```python
from build123d import *

# Parameters (mm, degrees)
F1_DEPTH  = 4
F0_W      = 107
F0_H      = 2.5
F2_DEPTH  = 33
F3_W      = 20
F3_H      = 19.215
F3_R      = 2.2232187412
F4_DEPTH  = 2
F6_D      = 4
F6_DEPTH  = 12
F6_TIP    = 1.2017212381
F7_D      = 4
F8_DEPTH  = 10
F9_F1_R   = 1.9313708499
F9_F2_R   = 1.9313708499
F10_W     = 15
F10_H     = 10
F11_DEPTH = 11.3
F0_W_2    = 2.4193752706
F0_H_2    = 9.5048956573
F0_W_3    = 2.649404496
F0_H_3    = 10.744664818
F12_DEPTH = 25
F13_R     = 1.2071067812


with BuildPart() as f1:
    # F0 (on Top) → F1 (new body)
    with BuildSketch(Plane.XY):
        Polygon((-53.5, -35), (53.5, -35), (53.5, -5.4848068394), (53.5, 5.2598579787), (53.5, 35), (-53.5, 35), (-53.5, 25.9394217283), (-53.5, 16.434526071), (-53.5, -16.434526071), (-53.5, -25.9394217283), align=None)
        with BuildLine():
            Line((38.5, 24), (38.5, -24))
            Line((38.5, -24), (7.5, -24))
            ThreePointArc((7.5, -24), (1.5, -19), (-4.5, -24))
            Line((-4.5, -24), (-38.5, -24))
            Line((-38.5, -24), (-38.5, 24))
            Line((-38.5, 24), (-4.5, 24))
            ThreePointArc((-4.5, 24), (1.5, 19), (7.5, 24))
            Line((7.5, 24), (38.5, 24))
        make_face(mode=Mode.SUBTRACT)
    extrude(amount=F1_DEPTH)

    # F0 (on Top) → F2 (join)
    with BuildSketch(Plane.XY):
        with Locations((0, 36.25)):
            Rectangle(F0_W, F0_H)
        with Locations((0, -36.25)):
            Rectangle(F0_W, F0_H)
    extrude(amount=F2_DEPTH)

    # F3 (on face) → F4 (join)
    with BuildSketch(Plane.XY):
        with Locations((-37.3952314258, -44.6075)):
            Rectangle(F3_W, F3_H)
        with Locations((-37.3952314258, -41.215)):
            Circle(F3_R, mode=Mode.SUBTRACT)
        with Locations((37.3952314258, -44.6075)):
            Rectangle(F3_W, F3_H)
        with Locations((37.3952314258, -41.215)):
            Circle(F3_R, mode=Mode.SUBTRACT)
        with Locations((37.3952314258, 44.6075)):
            Rectangle(F3_W, F3_H)
        with Locations((37.3952314258, 41.215)):
            Circle(F3_R, mode=Mode.SUBTRACT)
        with Locations((-37.3952314258, 44.6075)):
            Rectangle(F3_W, F3_H)
        with Locations((-37.3952314258, 41.215)):
            Circle(F3_R, mode=Mode.SUBTRACT)
    extrude(amount=F4_DEPTH)

    # F6
    with Locations(Plane(origin=(0, 37.5, 0), x_dir=(-1, 0, 0), z_dir=(0, 1, 0))):
        with Locations((43.5, 23)):
            Hole(F6_D / 2, depth=F6_DEPTH)
            with Locations((0, 0, -(F6_DEPTH + F6_TIP / 2))):  # 118° drill point
                Cone(0, F6_D / 2, F6_TIP, mode=Mode.SUBTRACT)

    # F7 (through all)
    with Locations(Plane(origin=(0, 37.5, 0), x_dir=(-1, 0, 0), z_dir=(0, 1, 0))):
        with Locations((0, 16.522007063)):
            Hole(F7_D / 2)

    # F0 (on Top) → F8 (join)
    with BuildSketch(Plane.XY):
        with BuildLine():
            Line((7.5, -24), (38.5, -24))
            Line((38.5, -24), (38.5, 24))
            Line((38.5, 24), (7.5, 24))
            ThreePointArc((7.5, 24), (1.5, 19), (-4.5, 24))
            Line((-4.5, 24), (-38.5, 24))
            Line((-38.5, 24), (-38.5, -24))
            Line((-38.5, -24), (-4.5, -24))
            ThreePointArc((-4.5, -24), (1.5, -19), (7.5, -24))
        make_face()
    extrude(amount=F8_DEPTH)

    # F9: fillet of radius 1.9313708499 on 12 edges, made by hand

    # F9_f1
    f9_f1_edges = [f1.edges().sort_by_distance(p)[0] for p in [
        (0, -35, 4),
        (0, 35, 4),
        (1.5, 19, 4),
        (23, 24, 4),
        (38.5, 0, 4),
        (23, -24, 4),
        (1.5, -19, 4),
        (-21.5, -24, 4),
        (-38.5, 0, 4),
        (-21.5, 24, 4),
    ]]
    fillet(f9_f1_edges, radius=F9_F1_R)

    # F9_f2
    f9_f2_edges = [f1.edges().sort_by_distance(p)[0] for p in [
        (53.5, 0, 4),
        (-53.5, 0, 4),
        (-53.5, -34.4343145751, 4.5656854249),
        (-53.5, 34.4343145751, 4.5656854249),
        (53.5, 34.4343145751, 4.5656854249),
        (53.5, -34.4343145751, 4.5656854249),
    ]]
    fillet(f9_f2_edges, radius=F9_F2_R)

    # F10 (on face) → F11 (cut)
    with BuildSketch(Plane.XY):
        with Locations((-46.3137403131, 0)):
            Rectangle(F10_W, F10_H)
    extrude(amount=F11_DEPTH, mode=Mode.SUBTRACT)

    # F0 (on Top) → F12 (join)
    with BuildSketch(Plane.XY):
        with Locations((-54.7096876353, 21.1869738996)):
            Rectangle(F0_W_2, F0_H_2)
        with Locations((-54.7096876353, -21.1869738996)):
            Rectangle(F0_W_2, F0_H_2)
        with Locations((54.824702248, -0.1124744304)):
            Rectangle(F0_W_3, F0_H_3)
    extrude(amount=F12_DEPTH)

    # F13
    f13_edges = [f1.edges().sort_by_distance(p)[0] for p in [
        (-55.919375, 25.939422, 12.5),
        (-55.919375, 16.434526, 12.5),
        (-55.919375, 21.186974, 0),
        (-55.919375, 21.186974, 25),
        (-55.919375, -16.434526, 12.5),
        (-55.919375, -25.939422, 12.5),
        (-55.919375, -21.186974, 0),
        (-55.919375, -21.186974, 25),
        (56.149404, -5.484807, 12.5),
        (56.149404, 5.259858, 12.5),
        (56.149404, -0.112474, 0),
        (56.149404, -0.112474, 25),
    ]]
    fillet(f13_edges, radius=F13_R)


solid = f1.part
```
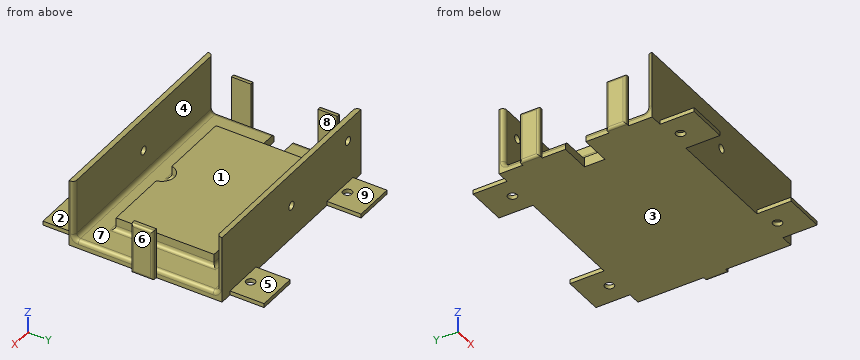
Model file for the job. Use its own axes, mm. Face numbers are marked on the shaded views. A direction names the side the tool comes from. Coordinates: 2 decimals unless noted, no trailing zeros. Loops run counter-clockwise (first coordinate to the right, second up) from the corner with the lowest first, then second, coordinate; pieces in that order, holes last. Notation, with made-up numbers: (-31.75, 58) -> (-25.75, 58) arc R28 cw to (-25.75, 85) -> close; hole circle Ø1 at (27, 40). An arc over 180 degrees is marked (long way). Answer as a JSON object with one key per item and string values.
Q1. Cut at C-C (x = 44). List the corners of the cut face in (y, z) (3 decimals), and give its area (3 significant figures).
Report:
{"outline": "(-54.215, 0) -> (54.215, 0) -> (54.215, 2) -> (37.5, 2) -> (37.5, 33) -> (35, 33) -> (35, 5.931) arc R1.931 cw to (33.069, 4) -> (-33.069, 4) arc R1.931 cw to (-35, 5.931) -> (-35, 33) -> (-37.5, 33) -> (-37.5, 2) -> (-54.215, 2) -> close", "area": "513 mm2"}
Q2. Cut at B-B (y = -11). List the corners of the cut face in (x, z).
Report:
{"outline": "(-53.5, 0) -> (53.5, 0) -> (53.5, 2.07) arc R1.93 ccw to (51.57, 4) -> (40.43, 4) arc R1.93 cw to (38.5, 5.93) -> (38.5, 10) -> (-38.5, 10) -> (-38.5, 5.93) arc R1.93 cw to (-40.43, 4) -> (-51.57, 4) arc R1.93 ccw to (-53.5, 2.07) -> close"}
Q3. Cut at A-A (x = -43.5). List the corners of the cut face in (y, z) (3 decimals), and give its area (3 significant figures).
Report:
{"outline": "(-54.215, 0) -> (-5, 0) -> (-5, 4) -> (-33.069, 4) arc R1.931 cw to (-35, 5.931) -> (-35, 33) -> (-37.5, 33) -> (-37.5, 2) -> (-54.215, 2) -> close; (5, 0) -> (54.215, 0) -> (54.215, 2) -> (37.5, 2) -> (37.5, 21) -> (35, 21) -> (35, 5.931) arc R1.931 cw to (33.069, 4) -> (5, 4) -> close; (35, 25) -> (37.5, 25) -> (37.5, 33) -> (35, 33) -> close", "area": "463 mm2"}
Q4. 3-axis set-ups, long thin cutter, end or side, ignore diameter. For the marked faces 1, 2, 3, 4 and 5: which of +Z, -Z, +X, -X, +Y, -Y reach the whole face in a straight line?
Report:
{"face 1": "+Z", "face 2": "+Z, +X, -X, -Y", "face 3": "-Z, +X, -X, +Y, -Y", "face 4": "+Z, +X, -X", "face 5": "+Z, +X, -X, +Y"}
Q5. Pull direction X, two halves, no side cores. Call the marked faces 6, 7, 8 and 9: released by +X, released by -X, zero draft, split by the parting line, or undercut.
Report:
{"face 6": "released by +X", "face 7": "undercut", "face 8": "undercut", "face 9": "zero draft"}
Q6. Cut at D-D (y = -31). List the corners of the cut face in (x, z), and give its area (3 significant figures).
Report:
{"outline": "(-53.5, 0) -> (53.5, 0) -> (53.5, 2.07) arc R1.93 ccw to (51.57, 4) -> (-51.57, 4) arc R1.93 ccw to (-53.5, 2.07) -> close", "area": "426 mm2"}
Q7. Probe probe 1 along Y at (x, z) = (-38.5, 11.5); probe 2 along X at (y, z) = (-17.5, 9); probe 3 along Y at (x, z) = (-1, 9.5). List the from-to ranges inside material, lowest first.
Report:
{"probe 1": "y = -37.5 to -35, 35 to 37.5", "probe 2": "x = -55.91 to -53.5, -38.5 to 38.5", "probe 3": "y = -37.5 to -35, -19.54 to 19.54, 35 to 37.5"}
Q8. Flat gauge pins, fed straight in: P1, Ø3.5, axis at x = 37.4, y = 41.22, coming from the +Z side; P2, Ø13.5, axis at x = -4.5, z = 17.5, coming from the +Y side; P3, Ø1.5, axis at x = -1.5, z = 19.5, coming from the -Y side; P4, Ø6, axis at x = 37.4, y = -41.22, coming from the +Z side. Where does each tip first touch, or does it go through?
Report:
{"P1": "passes through", "P2": "stops at y = 37.5", "P3": "stops at y = -37.5", "P4": "stops at z = 2"}
